```python
from build123d import *

# Parameters (mm, degrees)
SKETCH1_R           = 76.2
SKETCH1_R_2         = 1.3589
SKETCH1_R_3         = 4.9022
SKETCH1_R_4         = 2.38125
BOSS_EXTRUDE1_DEPTH = 6.35
SKETCH2_R           = 76.2
SKETCH2_R_2         = 74.041
CUT_EXTRUDE1_DEPTH  = 3.175
CUT_EXTRUDE2_START  = -3.175
CUT_EXTRUDE2_DEPTH  = 3.556


with BuildPart() as part:
    # Sketch1 → Boss-Extrude1 (new body)
    with BuildSketch(Plane(origin=(0, 0, 0), x_dir=(1, 0, 0), z_dir=(0, 1, 0))):
        Circle(SKETCH1_R)
        with Locations((26.940768363, 26.940768363)):
            Circle(SKETCH1_R_2, mode=Mode.SUBTRACT)
        with Locations((26.940768363, -26.940768363)):
            Circle(SKETCH1_R_2, mode=Mode.SUBTRACT)
        with Locations((-26.940768363, 26.940768363)):
            Circle(SKETCH1_R_2, mode=Mode.SUBTRACT)
        with Locations((43.18, 0)):
            Circle(SKETCH1_R_3, mode=Mode.SUBTRACT)
        with Locations((-43.18, 0)):
            Circle(SKETCH1_R_3, mode=Mode.SUBTRACT)
        with Locations((-13.470384182, 13.470384182)):
            Circle(SKETCH1_R_4, mode=Mode.SUBTRACT)
        with Locations((-26.940768363, -26.940768363)):
            Circle(SKETCH1_R_2, mode=Mode.SUBTRACT)
    extrude(amount=BOSS_EXTRUDE1_DEPTH)

    # Sketch2 → Cut-Extrude1 (cut)
    with BuildSketch(Plane.XZ):
        Circle(SKETCH2_R)
        Circle(SKETCH2_R_2, mode=Mode.SUBTRACT)
    extrude(amount=-CUT_EXTRUDE1_DEPTH, mode=Mode.SUBTRACT)

    # Sketch3 → Cut-Extrude2 (cut)
    with BuildSketch(Plane(origin=(0, 6.35, 0), x_dir=(1, 0, 0), z_dir=(0, 1, 0)).offset(CUT_EXTRUDE2_START)):
        with BuildLine():
            Line((3.2385, 34.798), (3.2385, 13.97))
            ThreePointArc((3.2385, 13.97), (0, 10.7315), (-3.2385, 13.97))
            Line((-3.2385, 13.97), (-3.2385, 34.798))
            ThreePointArc((-3.2385, 34.798), (0, 38.0365), (3.2385, 34.798))
        make_face()
        with BuildLine():
            Line((3.2385, -34.798), (3.2385, -13.97))
            ThreePointArc((3.2385, -13.97), (0, -10.7315), (-3.2385, -13.97))
            Line((-3.2385, -13.97), (-3.2385, -34.798))
            ThreePointArc((-3.2385, -34.798), (0, -38.0365), (3.2385, -34.798))
        make_face()
    extrude(amount=-CUT_EXTRUDE2_DEPTH, mode=Mode.SUBTRACT)


solid = part.part
```
Work out the finished part from the listing and answer in its coordinate system (mm). A direction names the side the tool comes from. Coordinates: 2 decimals unless noted, no trailing zeros. Loops run counter-clockwise (first coordinate to the right, second up) from the corner with the lowest first, then second, coordinate; pieces in that order, holes last. Notation, with made-up numbers: M 52.5,34.25 L 110.5,34.25 A12 ccw 110.5,42.25 Z; hole C 4,23.25 d2. An arc over 180 degrees is marked long. Use CSV: the item, a comma, the result in double quotes. Start each with the question number.
(1) For a pull along Z with two mould halves and no side action, classify faces 3 (the face through (-1, 6.35, -1)), 4 (the face through (-16.05, 1.57, -72.28)), 5 (the face through (0.071, 1.61, -10.732)) as +Z half, -Z half, draft (parallel to the pull), parting line (faces both ways), or undercut.
(2) Find section D-D, the plane y = 4.25. Give the vertices of the cut face in (x, z).
(3) Consider line 1 (X direction, y = 6, z = -26); line 2 (X direction, y = 2.75, z = 19); line 3 (X direction, y = 2, z = -28.5). Determine where each line is inside the solid, lowest interval first.
(4) Find section A-A, the plane x = 43.18. Give the vertices of the cut face in (y, z) (3 decimals).
(5) For faces 1 (the face through (0, 3.175, -25)), 2 (the face through (-1, 0, -1)), determine the directions among +Z, -Z, +X, -X, +Y, -Y from which every point of the face is accessible in a straight line to the end or side of a thin tool.
(6) Given pin 1 Ø3 at (x, y) = (-16, 2) entering from +Z; pin 2 Ø3.5 at (y, z) = (1, 25) entering from -X; pin 3 Ø3 at (x, z) = (1.5, -25) entering from -Y (3 decimals), each flat-ended and moving along its own axis, determine where each tip first touches the part or whether it passes through.
Recorded:
1,face 3,"draft"
1,face 4,"parting line"
1,face 5,"undercut"
2,outline,"C 0,0 d152.4; hole C -43.18,0 d9.8; hole C -26.94,-26.94 d2.72; hole C -26.94,26.94 d2.72; hole C -13.47,-13.47 d4.76; hole C 26.94,-26.94 d2.72; hole C 26.94,26.94 d2.72; hole C 43.18,0 d9.8"
3,line 1,"x = -71.63 to -27.92, -25.96 to 25.96, 27.92 to 71.63"
3,line 2,"x = -71.56 to -3.24, 3.24 to 71.56"
3,line 3,"x = -68.34 to -3.24, 3.24 to 68.34"
4,outline,"M 0,-60.146 L 3.175,-60.146 L 3.175,-62.785 L 6.35,-62.785 L 6.35,-4.902 L 0,-4.902 Z; M 0,4.902 L 6.35,4.902 L 6.35,62.785 L 3.175,62.785 L 3.175,60.146 L 0,60.146 Z"
5,face 1,"-Y"
5,face 2,"+Z, -Z, +X, -X, -Y"
6,pin 1,"stops at z = 74.7"
6,pin 2,"stops at x = -70.3"
6,pin 3,"stops at y = 3.175"
